Geometry check sheet. Reference: drawing and pictorial views, mm from the part's lowest x, y, z. A direction names the side the tool comes from. Give positions to 0.01 mm unless a question says otherwise; leave off trailing zeros. Loops run counter-clockwise (first coordinate to the right, second up) from the corner with the lowest first, then second, coordinate; pieces in that order, holes last. Notation, with made-up numbers: (55, -38) -> (90, -38) arc R23 ccw to (90, -30) -> close; hole circle Ø1 at (-34.75, -27). An arc over 180 degrees is marked (long way). Write each question's results on one line, items separated by ' | '. Start each with the question number.
1. Material ranges on L1, parallel to Y at x = 7, z = 0.5; L2, parallel to Y at x = 22, z = 1.2; L3, parallel to Y at x = 37, z = 0.6, recorded low to high. Write a range as from..to.
2. Cross-section at A-A on x = 37. Record the boundary of the cut face in (y, z) (3 decimals), and give its area (3 significant figures).
3. Tool access check on the marked faces 1 and 2. Record the directions out of +Z, -Z, +X, -X, +Y, -Y that give a thin tool (end or side, any length) a straight path to the whole face; none if there is none.
4. Cross-section at D-D on z = 2.8. Record the boundary of the cut face in (x, y) (3 decimals).
5. Gauge pin test, flat ends, axial feed: pin 1 Ø4 at (x, y) = (5.5, 24) entering from +Z; pin 2 Ø2.5 at (x, y) = (22, 5.5) entering from +Z. Record the tip position at first contact, or that the pin passes through.
6. Cross-section at C-C on y = 14.5. Record the boundary of the cut face in (x, z) (3 decimals), and give its area (3 significant figures).
7. Cross-section at B-B on y = 5.5. Record the boundary of the cut face in (x, z) (3 decimals).
8. Mould release check, pull along X, two halves, no side actions. Record for the marked faces 3, 4 and 5: +X half, -X half, draft (parallel to the pull), parting line (faces both ways), or undercut.
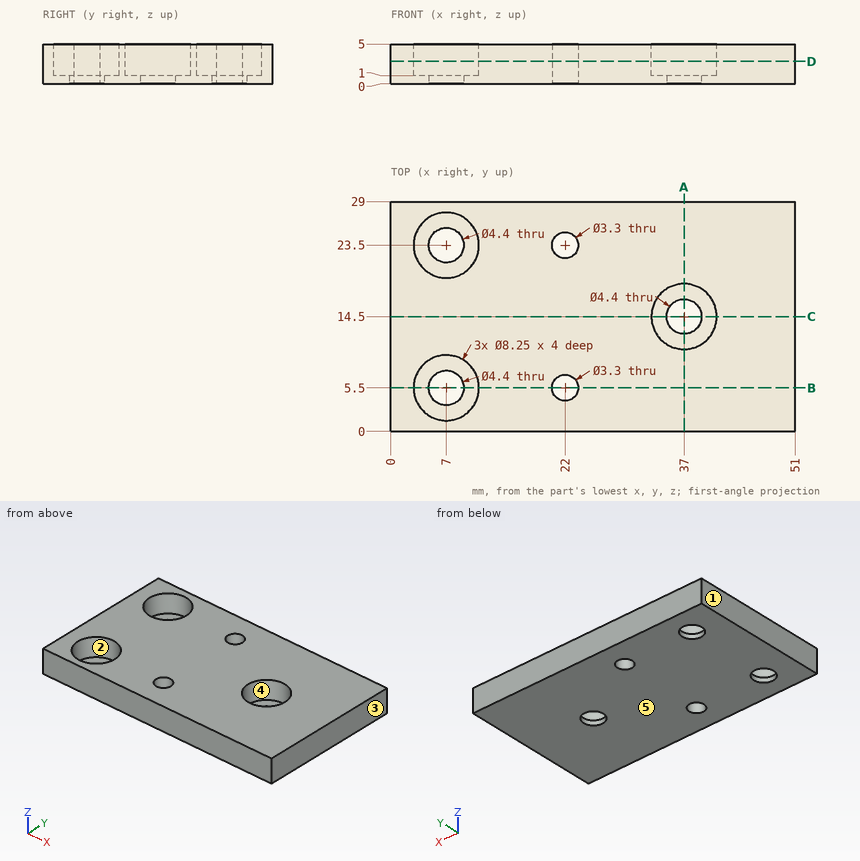
Geometry says:
1) L1: 0..3.3, 7.7..21.3, 25.7..29 | L2: 0..3.85, 7.15..21.85, 25.15..29 | L3: 0..12.3, 16.7..29
2) outline: (0, 0) -> (12.3, 0) -> (12.3, 1) -> (10.375, 1) -> (10.375, 5) -> (0, 5) -> close; (16.7, 0) -> (29, 0) -> (29, 5) -> (18.625, 5) -> (18.625, 1) -> (16.7, 1) -> close | area: 108 mm^2
3) face 1: +Z, -Z, -X, +Y, -Y | face 2: +Z
4) outline: (0, 0) -> (51, 0) -> (51, 29) -> (0, 29) -> close; hole circle Ø8.25 at (7, 5.5); hole circle Ø8.25 at (7, 23.5); hole circle Ø3.3 at (22, 5.5); hole circle Ø3.3 at (22, 23.5); hole circle Ø8.25 at (37, 14.5)
5) pin 1: z = 1 | pin 2: through
6) outline: (0, 0) -> (34.8, 0) -> (34.8, 1) -> (32.875, 1) -> (32.875, 5) -> (0, 5) -> close; (39.2, 0) -> (51, 0) -> (51, 5) -> (41.125, 5) -> (41.125, 1) -> (39.2, 1) -> close | area: 218 mm^2
7) outline: (0, 0) -> (4.8, 0) -> (4.8, 1) -> (2.875, 1) -> (2.875, 5) -> (0, 5) -> close; (9.2, 0) -> (20.35, 0) -> (20.35, 5) -> (11.125, 5) -> (11.125, 1) -> (9.2, 1) -> close; (23.65, 0) -> (51, 0) -> (51, 5) -> (23.65, 5) -> close
8) face 3: +X half | face 4: undercut | face 5: draft
